from build123d import *

# Parameters (mm, degrees)
SKETCH3_R                               = 14.325
BOSS_EXTRUDE3_DEPTH                     = 20
CBORE_FOR_M5_HEX_HEAD_BOLT1_D           = 5.5
CBORE_FOR_M5_HEX_HEAD_BOLT1_DEPTH       = 10
CBORE_FOR_M5_HEX_HEAD_BOLT1_CBORE_D     = 12.24
CBORE_FOR_M5_HEX_HEAD_BOLT1_CBORE_DEPTH = 3.58
FILLET1_R                               = 2


with BuildPart() as part:
    # Sketch3 → Boss-Extrude3 (new body)
    with BuildSketch(Plane.XY):
        with BuildLine():
            ThreePointArc((35, 5), (0, 40), (-35, 5))
            Line((-35, 5), (-50, 5))
            Line((-50, 5), (-50, -5))
            Line((-50, -5), (50, -5))
            Line((50, -5), (50, 5))
            Line((50, 5), (35, 5))
        make_face()
        with Locations((0, 19.325)):
            Circle(SKETCH3_R, mode=Mode.SUBTRACT)
    extrude(amount=BOSS_EXTRUDE3_DEPTH)

    # CBORE for M5 Hex Head Bolt1
    with Locations(Plane(origin=(0, 5, 0), x_dir=(1, 0, 0), z_dir=(0, 1, 0))):
        with Locations((-42.5, -10), (42.5, -10)):
            CounterBoreHole(CBORE_FOR_M5_HEX_HEAD_BOLT1_D / 2, CBORE_FOR_M5_HEX_HEAD_BOLT1_CBORE_D / 2, CBORE_FOR_M5_HEX_HEAD_BOLT1_CBORE_DEPTH, depth=CBORE_FOR_M5_HEX_HEAD_BOLT1_DEPTH)

    # Fillet1
    fillet1_edges = [part.edges().sort_by_distance(p)[0] for p in [
        (50, 0, 0),
        (-50, 0, 0),
        (50, 0, 20),
        (-50, 0, 20),
    ]]
    fillet(fillet1_edges, radius=FILLET1_R)


solid = part.part
Input: part model. Units: mm. Frame: model coordinates. A direction names the side the tool comes from. Coordinates: 2 decimals unless noted, no trailing zeros. Order: outer loops, then holes, each group sorted by start corner. A loop starts at its lowest first (then second) coordinate and runs counter-clockwise, first axis right, second up.
1. Contact query for flat-ended pins moving along their axis: P1, Ø1, axis at y = 22, z = 9, coming from the -X side; P2, Ø6, axis at x = 41.5, z = 9.5, coming from the +Y side; P3, Ø8, axis at y = 14, z = 16.5, coming from the -X side. Output: stop coordinate, or through.
Checked values:
P1: stops at x = -30.87
P2: stops at y = 1.42
P3: stops at x = -34.64
2. Cut plane B-B, the plane y = 0.5. Return loops of the section in (x, z), plus the area to 3 significant figures.
Checked values:
outline: (-50, 2) arc R2 ccw to (-48, 0) - (48, 0) arc R2 ccw to (50, 2) - (50, 18) arc R2 ccw to (48, 20) - (-48, 20) arc R2 ccw to (-50, 18) - close; hole circle Ø5.5 at (-42.5, 10); hole circle Ø5.5 at (42.5, 10)
area: 1,950 mm2
3. Draft query along Z for faces 1 (the flat face through (-1, -5, 10)), 2 (the flat face through (-1, 3, 0)), 3 (the cylindrical face through (-39.753, -1.835, 9.879)). Return one class per face: +Z half, -Z half, draft (parallel to the pull), parting line (faces both ways), or undercut.
Checked values:
face 1: draft
face 2: -Z half
face 3: undercut
4. Access query for faces 4 (the flat face through (-42, 5, 3)), 5 (the flat face through (49, 5, 10)), 6 (the flat face through (-1, 3, 20)), 7 (the cylindrical face through (49.4, 0.07, 0.57)), 8 (the flat face through (-39.9, 1.42, 11.3)). Directions: +Z, -Z, +X, -X, +Y, -Y. A direction counts if a zero-diameter tool reaches every point of the face in a straight line with its end or side. Return the directions, or none.
Checked values:
face 4: +Z, -Z, -X, +Y
face 5: +Z, -Z, +X, +Y
face 6: +Z, +X, -X, +Y, -Y
face 7: -Z, +X, +Y, -Y
face 8: +Y
5. Ray query, line 1 along Y through (x, z) = (0, 8.5); line 2 along X through (y, z) = (0, 10); line 3 along Z through (x, y) = (42.5, 0). Return the intervals inside material, ascending.
Checked values:
line 1: y = -5 to 5, 33.65 to 40
line 2: x = -50 to -45.25, -39.75 to 39.75, 45.25 to 50
line 3: z = 0 to 7.25, 12.75 to 20
6. Cut plane C-C, the plane z = 10. Return loops of the section in (x, y) (3 decimals).
Checked values:
outline: (-50, -5) - (-45.25, -5) - (-45.25, 1.42) - (-48.62, 1.42) - (-48.62, 5) - (-50, 5) - close; (-39.75, -5) - (39.75, -5) - (39.75, 1.42) - (36.38, 1.42) - (36.38, 5) - (35, 5) arc R35 ccw to (-35, 5) - (-36.38, 5) - (-36.38, 1.42) - (-39.75, 1.42) - close; (45.25, -5) - (50, -5) - (50, 5) - (48.62, 5) - (48.62, 1.42) - (45.25, 1.42) - close; hole circle Ø28.65 at (0, 19.325)
7. Cut plane A-A, the plane x = 42.5. Return loops of the section in (y, z).
Checked values:
outline: (-5, 0) - (5, 0) - (5, 3.88) - (1.42, 3.88) - (1.42, 7.25) - (-5, 7.25) - close; (-5, 12.75) - (1.42, 12.75) - (1.42, 16.12) - (5, 16.12) - (5, 20) - (-5, 20) - close
8. Cut plane D-D, the plane x = 0. Return loops of the section in (y, z), plus the area to 3 significant figures.
Checked values:
outline: (-5, 0) - (5, 0) - (5, 20) - (-5, 20) - close; (33.65, 0) - (40, 0) - (40, 20) - (33.65, 20) - close
area: 327 mm2
